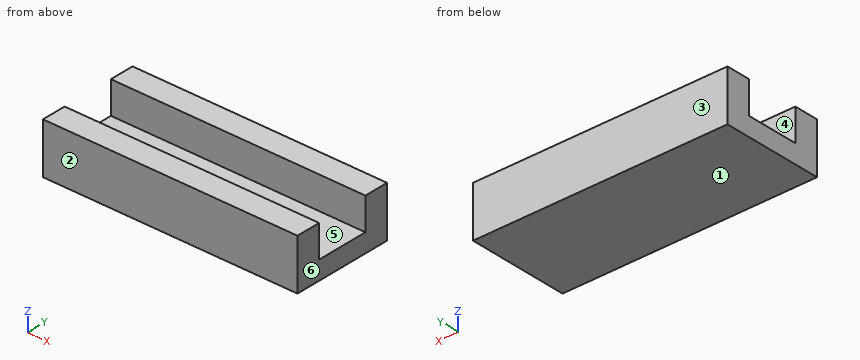
from build123d import *

# Parameters (mm, degrees)
F0_W     = 150
F0_H     = 14.5
F1_DEPTH = 30
F0_H_2   = 31
F2_DEPTH = 11
F3_DEPTH = 30


with BuildPart() as f1:
    # F0 (on Top) → F1 (new body)
    with BuildSketch(Plane.XY):
        with Locations((0, -22.75)):
            Rectangle(F0_W, F0_H)
    extrude(amount=F1_DEPTH)



with BuildPart() as f1b:
    # F0 (on Top) → F1, piece 2 (new body)
    with BuildSketch(Plane.XY):
        with Locations((0, 22.75)):
            Rectangle(F0_W, F0_H)
    extrude(amount=F1_DEPTH)


with BuildPart() as f1_1:
    add(f1.part)

    add(f1b.part)  # F2 merges F1b
    # F0 (on Top) → F2 (join)
    with BuildSketch(Plane.XY):
        Rectangle(F0_W, F0_H_2)
    extrude(amount=F2_DEPTH)

    # F0 (on Top) → F3 (join)
    with BuildSketch(Plane.XY):
        with Locations((0, 22.75)):
            Rectangle(F0_W, F0_H)
    extrude(amount=F3_DEPTH)


solid = f1_1.part
Geometry check sheet. Reference: the model listing, model coordinates, mm. Face numbers are marked on the shaded views. A direction names the side the tool comes from. Give positions to 0.01 mm unless a question says otherwise; leave off trailing zeros. Loops run counter-clockwise (first coordinate to the right, second up) from the corner with the lowest first, then second, coordinate; pieces in that order, holes last.
(1) Set-up check for the marked faces 5 and 6: record each of +Z, -Z, +X, -X, +Y, -Y from which the full face is reachable in a straight line by a thin tool's end or side.
From the geometry:
face 5: +Z, +X, -X
face 6: +Z, -Z, +X, +Y, -Y
(2) Section check B-B on x = 10. Record the cut outline in (y, z).
From the geometry:
outline: (-30, 0) - (30, 0) - (30, 30) - (15.5, 30) - (15.5, 11) - (-15.5, 11) - (-15.5, 30) - (-30, 30) - close
(3) Thickness scan on L1, parallel to Y at x = -47, z = 21.5; L2, parallel to Z at x = 67, y = -9. Record the ranges inside material, lowest first.
From the geometry:
L1: y = -30 to -15.5, 15.5 to 30
L2: z = 0 to 11
(4) Section check C-C on y = -8.5. Record the cut outline in (x, z).
From the geometry:
outline: (-75, 0) - (75, 0) - (75, 11) - (-75, 11) - close
(5) Depth check by flat-ended pin: pin 1 Ø10 at (y, z) = (-8, 17) entering from +X; pin 2 Ø15.5 at (x, y) = (-31.5, 5.5) entering from +Z. Enter the tip coordinate at first touch or a pass-through.
From the geometry:
pin 1: passes through
pin 2: stops at z = 11
(6) Release check for a two-part mould opening along Y. For the marked faces 1, 2, 3 and 4 record: released by +Y, released by -Y, zero draft, split by the parting line, or undercut.
From the geometry:
face 1: zero draft
face 2: released by -Y
face 3: released by +Y
face 4: undercut
(7) Section check A-A on z = 19. Record the cut outline in (x, y), then the cut area to 3 significant figures.
From the geometry:
outline: (-75, -30) - (75, -30) - (75, -15.5) - (-75, -15.5) - close; (-75, 15.5) - (75, 15.5) - (75, 30) - (-75, 30) - close
area: 4,350 mm2
